Geometry: final body of the model. Coordinates: model frame, mm. A direction names the side the tool comes from. Give positions to 0.01 mm unless a question says otherwise; leave off trailing zeros. Write each loop counter-clockwise with the first axis right and the second up, starting at its lowest first coordinate (ties: lowest second). Pieces come first, ordered by that corner, then holes.
Q1. Cut plane D-D on z = 27.5. Return the cut outline in (x, y) (3 decimals), plus the area to 3 significant figures.
Q2. Line query: L1, parallel to Z at x = 0, y = 10.6 (3 decimals); L2, parallel to Y at x = 0, z = 36 (3 decimals); L3, parallel to Z at x = 0, y = 11.3. Output: solid intervals per line, ascending.
Q3. Draft query along Y for faces 4 (the face through (-11.732, 4.864, 23.017)), 5 (the face through (0.132, -10.888, 34.747)), 6 (the face through (0, 0, 25.4)). Return one class per face: pulls with the +Y half, pulls with the -Y half, needs draft (parallel to the pull), parting line crosses it, or undercut.
Q4. Cut plane A-A on x = 1.25. Count the separate pieces of the cut face and the enclosed holes in it, plus the area to 3 significant figures.
Q5. Cut plane B-B on z = 31.75. Return the cut outline in (x, y) (3 decimals).
Q6. Cut plane C-C on y = 0. Return the cut outline in (x, z) (3 decimals).
Q7. Reachability of faces 1 (the face through (0.4, 10.3, 9.5)), 2 (the face through (0, -9.525, 3)), 3 (the face through (9.085, 2.861, 31.839)) from +Z, -Z, +X, -X, +Y, -Y: full face, straight path, thin tool, end or side. Return the list, or none.
Q8. Pin query (flat end, axial travel): pin 1 (1.9 mm diameter, centred on x = 1.5, z = 7.5, fed in from +Y); pin 2 (5.5 mm diameter, centred on x = -3.5, y = 2.5, fed in from +Z); pin 3 (3 mm diameter, centred on y = -3.5, z = 14.5, fed in from +X). Return the tip coordinate at first contact, or that it passes through.
```python
from build123d import *

# Parameters (mm, degrees)
SKETCH1_R               = 12.7
BOSS_EXTRUDE1_DEPTH     = 38.1
CUT_EXTRUDE2_START      = -25.4000001
CUT_EXTRUDE2_DEPTH      = 25.4000001
CUT_EXTRUDE3_DEPTH      = 38.1
SKETCH4_R               = 9.525
CUT_EXTRUDE4_DEPTH      = 12.7
CUT_EXTRUDE5_DEPTH      = 11.1125
CUT_EXTRUDE5_DEPTH_BACK = 11.1125
SKETCH6_R               = 3.175
SKETCH7_R               = 3
CUT_EXTRUDE6_DEPTH      = 48.519048972


# Read off the part's stored shape, not the designer's step: Cut-Extrude2
with BuildPart() as part:
    # Sketch1 → Boss-Extrude1 (new body)
    with BuildSketch(Plane.XY):
        with Locations(Location((0, 0, 0), (0, 0, 180))):
            Circle(SKETCH1_R)
    extrude(amount=BOSS_EXTRUDE1_DEPTH)

    # Cut-Extrude2 outline → Cut-Extrude2 (cut)
    with BuildSketch(Plane(origin=(12.7, 0, 0), x_dir=(0, 0, -1), z_dir=(1, 0, 0)).offset(CUT_EXTRUDE2_START)):
        with BuildLine():
            Line((0, 9.525), (-6.35, 9.525))
            ThreePointArc((-6.35, 9.525), (-15.875, 0), (-6.35, -9.525))
            Line((-6.35, -9.525), (0, -9.525))
            Line((0, -9.525), (0, 9.525))
        make_face()
    extrude(amount=CUT_EXTRUDE2_DEPTH, mode=Mode.SUBTRACT)

    # Sketch3 → Cut-Extrude3 (cut)
    with BuildSketch(Plane(origin=(0, -12.7, 0), x_dir=(-1, 0, 0), z_dir=(0, -1, 0))):
        with BuildLine():
            ThreePointArc((-8.400260413, -5.241151589), (-4.934653756, -1.443317517), (0, 0))
            Line((0, 0), (-8.400260413, 0))
            Line((-8.400260413, 0), (-8.400260413, -5.241151589))
        make_face()
        with BuildLine():
            Line((8.400260413, 0), (0.21470184, 0))
            ThreePointArc((0.21470184, 0), (4.954513337, -1.324965695), (8.400260413, -4.838962595))
            Line((8.400260413, -4.838962595), (8.400260413, 0))
        make_face()
    extrude(amount=-CUT_EXTRUDE3_DEPTH, mode=Mode.SUBTRACT)

    # Sketch4 → Cut-Extrude4 (cut)
    with BuildSketch(Plane.XY.offset(38.1)):
        Circle(SKETCH4_R)
    extrude(amount=-CUT_EXTRUDE4_DEPTH, mode=Mode.SUBTRACT)

    # Sketch6 → Cut-Extrude5 (cut, two sides: drawn at the far end of the back side and taken through both)
    with BuildSketch(Plane(origin=(0, 0, 0), x_dir=(1, 0, 0), z_dir=(0, 1, 0)).offset(-CUT_EXTRUDE5_DEPTH_BACK)):
        with Locations(Location((0, -6.35, 0), (0, 0, 180))):
            Circle(SKETCH6_R)
    extrude(amount=CUT_EXTRUDE5_DEPTH + CUT_EXTRUDE5_DEPTH_BACK, mode=Mode.SUBTRACT)

    # Sketch7 → Cut-Extrude6 (cut, through all)
    with BuildSketch(Plane(origin=(0, -12.7, 0), x_dir=(-1, 0, 0), z_dir=(0, -1, 0))):
        with Locations(Location((0, -31.75, 0), (0, 0, 90))):
            Circle(SKETCH7_R)
    extrude(amount=-CUT_EXTRUDE6_DEPTH, mode=Mode.SUBTRACT)


solid = part.part
```
Data:
1. outline: circle Ø25.4 at (0, 0); hole circle Ø19.05 at (0, 0)
1. area: 222 mm2
2. L1: z = 0 to 3.175, 9.525 to 28.75, 34.75 to 38.1
2. L2: y = -12.7 to -9.525, 9.525 to 12.7
2. L3: z = 0 to 28.75, 34.75 to 38.1
3. face 4: parting line crosses it
3. face 5: needs draft
3. face 6: undercut
4. separate pieces: 3
4. enclosed holes: 0
4. area: 405 mm2
5. outline: (-3, -12.341) - (-3, -9.04) arc R9.525 cw to (-3, 9.04) - (-3, 12.341) arc R12.7 ccw to start; (3, -12.341) arc R12.7 ccw to (3, 12.341) - (3, 9.04) arc R9.525 cw to (3, -9.04) - close
6. outline: (-12.7, 15.875) - (12.7, 15.875) - (12.7, 38.1) - (9.525, 38.1) - (9.525, 25.4) - (-9.525, 25.4) - (-9.525, 38.1) - (-12.7, 38.1) - close
7. face 1: none
7. face 2: -Z, +X, -X
7. face 3: +Z
8. pin 1: stops at y = 12.69
8. pin 2: stops at z = 25.4
8. pin 3: stops at x = 12.46
